```python
from build123d import *

# Parameters (mm, degrees)
SALIENTE_EXTRUIR1_DEPTH      = 10
SALIENTE_EXTRUIR1_DEPTH_BACK = 10


with BuildPart() as part:
    # Croquis1 → Revoluci_n1 (revolve)
    with BuildSketch(Plane.XY, mode=Mode.PRIVATE) as revoluci_n1_sk:
        Polygon((0, 0), (3.75, 0), (3.75, 7.5), (25, 7.5), (25, 12.252764843), (0, 12.252764843), align=None)
    revolve(revoluci_n1_sk.sketch.rotate(Axis((0, 0, 0), (0, 1, 0)), 90), axis=Axis((0, 0, 0), (0, 1, 0)))

    # Croquis2 → Saliente-Extruir1 (add, two sides: drawn at the far end of the back side and taken through both)
    with BuildSketch(Plane.XY.offset(-SALIENTE_EXTRUIR1_DEPTH_BACK)):
        with BuildLine():
            Line((-1.941142838, 26.99720854), (-2.588190451, 29.412023106))
            ThreePointArc((-2.588190451, 29.412023106), (0, 9.752764843), (2.588190451, 29.412023106))
            Line((2.588190451, 29.412023106), (1.941142838, 26.99720854))
            ThreePointArc((1.941142838, 26.99720854), (0, 12.252764843), (-1.941142838, 26.99720854))
        make_face()
    extrude(amount=SALIENTE_EXTRUIR1_DEPTH + SALIENTE_EXTRUIR1_DEPTH_BACK)


solid = part.part
```
Here's how the part is built. I have some questions about the finished solid (model axes, mm). A direction names the side the tool comes from. Coordinates: 2 decimals unless noted, no trailing zeros. Order: outer loops, then holes, each group sorted by start corner. A loop starts at its lowest first (then second) coordinate and runs counter-clockwise, first axis right, second up. Notation, with made-up numbers: M -29.75,30.25 L 18.25,30.25 A24 ccw 18.25,65.25 Z; hole C 8,82 d3. An arc over 180 degrees is marked long. Answer as a JSON object with one key per item and string values. Group by question number.
(1) For pin 1 (11 mm diameter, centred on x = 3, y = 18, fed in from +Z); pin 2 (10 mm diameter, centred on x = 9, z = 13.5, fed in from -Y); pin 3 (8 mm diameter, centred on x = -6, y = 18, fed in from -Z), each with a flat end and sliding along its axis, tell me the tip position at first contact or that it passes through.
(2) Which directions (+Z, -Z, +X, -X, +Y, -Y) give clear straight access to the entire face, cutting with the end or side of a thin tool? Please do faces 1 (the face through (-2.26, 28.19, -0.14)), 2 (the face through (-3.16, 3.8, -2.02)), 3 (the face through (-8, 20, 10)).
(3) Suppose I cut it at D-D, the plane z = 0. Please give me the cut outline in (x, y).
(4) Suppose I cut it at B-B, the plane x = -9. Please give me the cut outline in (y, z), then the cut area to 3 significant figures.
(5) If we mould it in two halves opening along X, with no side actions, what happens to faces 4 (the face through (-7.509, 9.91, -23.846)), 5 (the face through (2.27, 28.22, -0.14)), 6 (the face through (0, 0, 0))? For each: released by +X, released by -X, zero draft, split by the parting line, or undercut.
(6) Suppose I cut it at A-A, the plane y = 21. Please give me the cut outline in (x, z), then the cut area to 3 significant figures.
(7) Suppose I cut it at C-C, the plane x = 1. Please give me the cut outline in (y, z), then the cut area to 3 significant figures.
(8) I need wall thicknesses on probe 1 along Y at (x, z) = (12, -19); probe 2 along Y at (x, z) = (3.5, -5.5); probe 3 along Z at (x, y) = (17, 11.75). Which ranges of each line are inside material? Lowest first, please.
Values found:
{
 "1": {"pin 1": "stops at z = 10", "pin 2": "stops at y = 7.5", "pin 3": "stops at z = -10"},
 "2": {"face 1": "+Z, -Z, +Y", "face 2": "-Y", "face 3": "+Z, +X, -X, +Y"},
 "3": {"outline": "M -25,7.5 L -3.75,7.5 L -3.75,0 L 3.75,0 L 3.75,7.5 L 25,7.5 L 25,12.25 L 6.61,12.25 A10 ccw 2.59,29.41 L 1.94,27 A7.5 cw long -1.94,27 L -2.59,29.41 A10 ccw -6.61,12.25 L -25,12.25 Z"},
 "4": {"outline": "M 7.5,-23.32 L 12.25,-23.32 L 12.25,23.32 L 7.5,23.32 Z; M 15.39,-10 L 24.11,-10 L 24.11,10 L 15.39,10 Z", "area": "396 mm^2"},
 "5": {"face 4": "split by the parting line", "face 5": "undercut", "face 6": "zero draft"},
 "6": {"outline": "M -9.92,-10 L -7.4,-10 L -7.4,10 L -9.92,10 Z; M 7.4,-10 L 9.92,-10 L 9.92,10 L 7.4,10 Z", "area": "101 mm^2"},
 "7": {"outline": "M 0,-3.61 L 7.5,-3.61 L 7.5,-24.98 L 12.25,-24.98 L 12.25,-10 L 12.32,-10 L 12.32,10 L 12.25,10 L 12.25,24.98 L 7.5,24.98 L 7.5,3.61 L 0,3.61 Z", "area": "293 mm^2"},
 "8": {"probe 1": "y = 7.5 to 12.25", "probe 2": "y = 7.5 to 13.12, 26.39 to 29.12", "probe 3": "z = -18.33 to 18.33"}
}
